Geometry: final body of the model. Coordinates: model frame, mm. A direction names the side the tool comes from. Coordinates: 2 decimals unless noted, no trailing zeros. Loops run counter-clockwise (first coordinate to the right, second up) from the corner with the lowest first, then second, coordinate; pieces in that order, holes last. Notation, with made-up numbers: (-21.5, 5) - (-11.5, 5) arc R17 ccw to (-11.5, 28) - close; hole circle Ø4 at (64.5, 24). An arc over 180 degrees is marked (long way). Answer in a Markdown table with one row per item.
from build123d import *

# Parameters (mm, degrees)
F1_DEPTH  = 125
F2_R      = 1.85
F3_DEPTH  = 4
F5_DEPTH  = 3
F7_R      = 6
F8_DEPTH  = 25
F10_R     = 6
F11_DEPTH = 25


with BuildPart() as f1:
    # F0 (on Front) → F1 (new body)
    with BuildSketch(Plane.XZ):
        Polygon((27.424138, 47.5), (-27.424138, 47.5), (-23.960036, 41.5), (23.960036, 41.5), align=None)
    extrude(amount=F1_DEPTH)

    # F2 (on face) → F3 (cut)
    with BuildSketch(Plane(origin=(0, 0, 41.5), x_dir=(1, 0, 0), z_dir=(0, 0, -1))):
        with BuildLine():
            ThreePointArc((-13.830018, 120), (-11.980018, 118.15), (-10.130018, 120))
            Line((-10.130018, 120), (-13.830018, 120))
        make_face()
        with BuildLine():
            Line((-13.830018, 120), (-10.130018, 120))
            ThreePointArc((-10.130018, 120), (-11.980018, 121.85), (-13.830018, 120))
        make_face()
        with Locations((11.980018, 120)):
            Circle(F2_R)
        with BuildLine():
            ThreePointArc((-13.830018, 23), (-11.980018, 21.15), (-10.130018, 23))
            Line((-10.130018, 23), (-13.830018, 23))
        make_face()
        with BuildLine():
            Line((-13.830018, 23), (-10.130018, 23))
            ThreePointArc((-10.130018, 23), (-11.980018, 24.85), (-13.830018, 23))
        make_face()
        with Locations((11.980018, 23)):
            Circle(F2_R)
    extrude(amount=-F3_DEPTH, mode=Mode.SUBTRACT)

    # F4 (on face) → F5 (join)
    with BuildSketch(Plane.XY.offset(47.5)):
        Polygon((-3.973212, -62.142442), (-9.196524, -68.068704), (0.688378, -67.934791), (6.248204, -60.093163), (1.484625, -60.093163), (7.940114, -49.645284), (-8.473853, -62.142442), align=None)
    extrude(amount=F5_DEPTH)

    # F7 (on face) → F8 (cut)
    with BuildSketch(Plane(origin=(-23.960036, 0, 41.5), x_dir=(0.866025, 0, 0.5), z_dir=(0.5, 0, -0.866025))):
        with Locations((0, 62.5)):
            Circle(F7_R)
    extrude(amount=F8_DEPTH, mode=Mode.SUBTRACT)

    # F10 (on face) → F11 (cut)
    with BuildSketch(Plane(origin=(23.960036, 0, 41.5), x_dir=(0.866025, 0, -0.5), z_dir=(0.5, 0, 0.866025))):
        with Locations((0, -62.5)):
            Circle(F10_R)
    extrude(amount=-F11_DEPTH, mode=Mode.SUBTRACT)


solid = f1.part
(1) Ray query, probe 1 along X at (y, z) = (-120, 42.3); probe 2 along X at (y, z) = (-120, 43.1); probe 3 along Z at (x, y) = (-14, -30). Return the intervals inside material, ascending.
Verdict:
| item | result |
|---|---|
| probe 1 | x = -24.42 to -13.83, -10.13 to 10.13, 13.83 to 24.42 |
| probe 2 | x = -24.88 to -13.83, -10.13 to 10.13, 13.83 to 24.88 |
| probe 3 | z = 41.5 to 47.5 |
(2) Cut plane B-B on x = -0.5. Output: boundary loops of the cut face in (y, z), then the cut area to 3 significant figures.
Verdict:
| item | result |
|---|---|
| outline | (-125, 41.5) - (0, 41.5) - (0, 47.5) - (-56.07, 47.5) - (-56.07, 50.5) - (-67.95, 50.5) - (-67.95, 47.5) - (-125, 47.5) - close |
| area | 786 mm² |
(3) Access query for faces 1 (the face through (-0.152, -55.806, 48.979)), 2 (the face through (-12.221, -24.834, 43.472)), 3 (the face through (4.67, -54.94, 48.98)), 4 (the face through (0, -62, 41.5)). Directions: +Z, -Z, +X, -X, +Y, -Y. A direction counts if a zero-diameter tool reaches every point of the face in a straight line with its end or side. Return the directions, or none.
Verdict:
| item | result |
|---|---|
| face 1 | +Z, -X, +Y |
| face 2 | -Z |
| face 3 | +Z, +X |
| face 4 | -Z, +X, -X, +Y, -Y |
(4) Pull-direction query (Y, two-part tool) for faces 5 (the face through (3.43, -64.07, 48.98)), 6 (the face through (4, -60.093, 49)), 7 (the face through (25.67, -61.62, 44.46)); classes: pulls with the +Y half, pulls with the -Y half, needs draft (parallel to the pull), parting line crosses it, or undercut.
Verdict:
| item | result |
|---|---|
| face 5 | pulls with the -Y half |
| face 6 | undercut |
| face 7 | needs draft |
(5) Cut plane D-D on y = -100. Output: boundary loops of the cut face in (x, z).
Verdict:
| item | result |
|---|---|
| outline | (-27.42, 47.5) - (-23.96, 41.5) - (23.96, 41.5) - (27.42, 47.5) - close |
(6) Cut plane C-C on x = 15. Output: boundary loops of the cut face in (y, z).
Verdict:
| item | result |
|---|---|
| outline | (-125, 41.5) - (0, 41.5) - (0, 47.5) - (-125, 47.5) - close |
(7) Cut plane A-A on y = -120. Output: boundary loops of the cut face in (x, z).
Verdict:
| item | result |
|---|---|
| outline | (-27.42, 47.5) - (-23.96, 41.5) - (-13.83, 41.5) - (-13.83, 45.5) - (-10.13, 45.5) - (-10.13, 41.5) - (10.13, 41.5) - (10.13, 45.5) - (13.83, 45.5) - (13.83, 41.5) - (23.96, 41.5) - (27.42, 47.5) - close |
(8) First-contact query: pin 1 Ø3 at (x, y) = (12.5, -120) entering from -Z; pin 2 Ø3 at (y, z) = (-76.5, 46.5) entering from +X; pin 3 Ø5 at (y, z) = (-42, 44) entering from +X; pin 4 Ø2.5 at (x, z) = (5, 49.5) entering from +Y. Flat tips, straight axial feed; report the tip coordinate or a pass-through.
Verdict:
| item | result |
|---|---|
| pin 1 | stops at z = 41.5 |
| pin 2 | stops at x = 27.42 |
| pin 3 | stops at x = 26.85 |
| pin 4 | stops at y = -50.93 |
